from build123d import *

# Parameters (mm, degrees)
SKIZZE1_W                            = 8
SKIZZE1_H                            = 30
AUFSATZ_LINEAR_AUSTRAGEN1_DEPTH      = 5
SKIZZE4_R                            = 1.6
SCHNITT_LINEAR_AUSTRAGEN4_DEPTH      = 18.720045147
VERRUNDUNG1_R                        = 5
SCHNITT_LINEAR_AUSTRAGEN5_DEPTH      = 18.720045147
SCHNITT_LINEAR_AUSTRAGEN5_DEPTH_BACK = 18.720045147
SKIZZE5_W                            = 0.8
SKIZZE5_H                            = 13


with BuildPart() as part:
    # Skizze1 → Aufsatz-Linear austragen1 (new, symmetric)
    with BuildSketch(Plane.XY):
        with Locations((-4, 0)):
            Rectangle(SKIZZE1_W, SKIZZE1_H)
    extrude(amount=AUFSATZ_LINEAR_AUSTRAGEN1_DEPTH, both=True)

    # Skizze4 → Schnitt-Linear austragen4 (cut, through all)
    with BuildSketch(Plane(origin=(0, 0, 0), x_dir=(0, 0, -1), z_dir=(1, 0, 0))):
        with Locations((0, 10.5)):
            Circle(SKIZZE4_R)
        with Locations((0, -10.5)):
            Circle(SKIZZE4_R)
    extrude(amount=-SCHNITT_LINEAR_AUSTRAGEN4_DEPTH, mode=Mode.SUBTRACT)

    # Verrundung1
    verrundung1_edges = [part.edges().sort_by_distance(p)[0] for p in [
        (-4, 15, 5),
        (-4, 15, -5),
        (-4, -15, 5),
        (-4, -15, -5),
    ]]
    fillet(verrundung1_edges, radius=VERRUNDUNG1_R - 0.0001)  # a hair under: the kernel refuses the full size

    # Skizze5 → Schnitt-Linear austragen5 (cut, two sides: drawn at the far end of the back side and taken through both)
    with BuildSketch(Plane.XY.offset(-SCHNITT_LINEAR_AUSTRAGEN5_DEPTH_BACK)):
        with Locations((-5.6, 0)):
            Rectangle(SKIZZE5_W, SKIZZE5_H)
    extrude(amount=SCHNITT_LINEAR_AUSTRAGEN5_DEPTH + SCHNITT_LINEAR_AUSTRAGEN5_DEPTH_BACK, mode=Mode.SUBTRACT)


solid = part.part
Design review of the part built by this model. Coordinates are the model's own, in mm. A direction names the side the tool comes from. Give positions to 0.01 mm unless a question says otherwise; leave off trailing zeros. Order: outer loops, then holes, each group sorted by start corner. A loop starts at its lowest first (then second) coordinate and runs counter-clockwise, first axis right, second up.
1. For pin 1 Ø1.5 at (x, z) = (-4.5, 3.5) entering from -Y; pin 2 Ø1 at (x, z) = (-1, -2.5) entering from +Y, all flat-tipped, find the tip position at first contact; note any pin that passes through.
Solution:
pin 1: stops at y = -14.18
pin 2: stops at y = 14.58
2. Tool access review of faces 1 (the cylindrical face through (-3.94, -12.06, 0.35)), 2 (the flat face through (-5.6, -6.5, -0.1)): name each direction out of +Z, -Z, +X, -X, +Y, -Y from which nothing blocks a thin tool from reaching the whole face with its end or side.
Solution:
face 1: +X, -X
face 2: +Z, -Z
3. Add section C-C, the plane z = -0.75. State the section outline as (x, y) points, then the cut area to 3 significant figures.
Solution:
outline: (-8, -14.94) - (0, -14.94) - (0, -11.91) - (-8, -11.91) - close; (-8, -9.09) - (0, -9.09) - (0, 9.09) - (-8, 9.09) - close; (-8, 11.91) - (0, 11.91) - (0, 14.94) - (-8, 14.94) - close; hole (-6, -6.5) - (-5.2, -6.5) - (-5.2, 6.5) - (-6, 6.5) - close
area: 183 mm2
4. Add section D-D, the plane z = -3.5. State the section outline as (x, y) points.
Solution:
outline: (-8, -13.57) - (0, -13.57) - (0, 13.57) - (-8, 13.57) - close; hole (-6, -6.5) - (-5.2, -6.5) - (-5.2, 6.5) - (-6, 6.5) - close
5. Add section B-B, the plane x = -6.75. State how many separate pieces and enclosed holes the cut face has, then the cut area to 3 significant figures.
Solution:
separate pieces: 1
enclosed holes: 2
area: 262 mm2
6. Mouldability with a two-part tool opening along X and no side actions: class faces 3 (the flat face through (-5.2, 0, 0)), 4 (the cylindrical face through (-4, 13, -4)), 5 (the flat face through (-5.6, 6.5, -0.1)), 6 (the flat face through (-8, 0, 0)) as +X half, -X half, draft (parallel to the pull), parting line (faces both ways), or undercut.
Solution:
face 3: undercut
face 4: draft
face 5: undercut
face 6: -X half
7. To check wall thickness, follow L1, parallel to Y at x = -4.5, z = 0; L2, parallel to X at y = 3.5, z = 4.75; L3, parallel to Y at x = -2, z = 1.25. State the ranges of each line that lie inside material, in increasing order.
Solution:
L1: y = -15 to -12.1, -8.9 to 8.9, 12.1 to 15
L2: x = -8 to -6, -5.2 to 0
L3: y = -14.84 to -11.5, -9.5 to 9.5, 11.5 to 14.84
8. Add section A-A, the plane y = -3.5. State the section outline as (x, z) points.
Solution:
outline: (-8, -5) - (-6, -5) - (-6, 5) - (-8, 5) - close; (-5.2, -5) - (0, -5) - (0, 5) - (-5.2, 5) - close
